```python
from build123d import *

# Parameters (mm, degrees)
F1_DEPTH = 7
F2_R     = 3.5
F3_DEPTH = 4
F5_DEPTH = 55
F7_DEPTH = 5


with BuildPart() as f1:
    # F0 (on Front) → F1 (new body)
    with BuildSketch(Plane.XZ):
        Polygon((12.5, 10), (0, 10), (-12.5, 10), (-12.5, 0.040646), (-12.5, -10), (12.5, -10), align=None)
    extrude(amount=F1_DEPTH)

    # F2 (on Front) → F3 (cut)
    with BuildSketch(Plane.XZ):
        Circle(F2_R)
    extrude(amount=F3_DEPTH, mode=Mode.SUBTRACT)

    # F4 (on face) → F5 (join)
    with BuildSketch(Plane.XZ.offset(7)):
        Polygon((2.5, 6.950472), (0, 6.950472), (-2.5, 6.950472), (-2.5, 1.950472), (2.5, 1.950472), align=None)
    extrude(amount=F5_DEPTH)

    # F6 (on face) → F7 (join)
    with BuildSketch(Plane.YZ.offset(2.5)):
        Polygon((-5.509801, -4.645343), (-18.229285, 1.950472), (-23.229285, 1.950472), (-5.509801, -8.645343), align=None)
    extrude(amount=-F7_DEPTH)


solid = f1.part
```
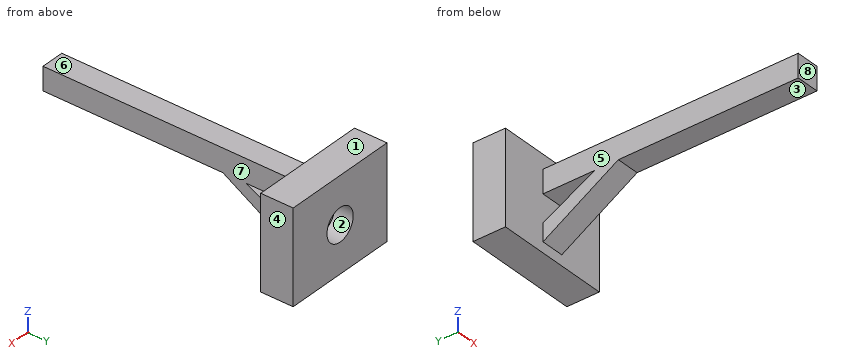
Design review of the part built by this model. Coordinates are the model's own, in mm. Face numbers are marked on the shaded views. A direction names the side the tool comes from. Give positions to 0.01 mm unless a question says otherwise; leave off trailing zeros. Loops run counter-clockwise (first coordinate to the right, second up) from the corner with the lowest first, then second, coordinate; pieces in that order, holes last. Notation, with made-up numbers: M 61.5,31 L 100.5,31 A7 ccw 100.5,37 Z; hole C -22,-22.75 d7. An arc over 180 degrees is marked long. Return JSON: item names as keys, results as strings. Group by question number.
Item 1: Mouldability with a two-part tool opening along Z and no side actions: class the marked faces 1, 2, 3 and 4 as released by +Z, released by -Z, zero draft, split by the parting line, or undercut.
Item 2: We need section C-C (x = 0). Give the boundary of the cut face in (y, z).
Item 3: We need section A-A (z = -1.5). Give the boundary of the cut face in (x, y), and give its area (3 significant figures).
Item 4: We need section D-D (y = -55.5). Give the boundary of the cut face in (x, z), and give its area (3 significant figures).
Item 5: Insertion check: pin 1 Ø7.5 at (y, z) = (-41.5, -3.5) entering from -X; pin 2 Ø2 at (x, y) = (1.5, -21.5) entering from -Z; pin 3 Ø10 at (x, y) = (4.5, -16.5) entering from +Z; pin 4 Ø1.5 at (x, y) = (1, -37) entering from -Z. Each pin has a flat end and moves straight along its axis. Give the tip position at first contact, or say it passes through.
Item 6: We need section B-B (y = -8). Give the boundary of the cut face in (x, z).
Item 7: For probe 1 along Z at (x, y) = (0, -2.55); probe 2 along Y at (x, z) = (7.5, 4.5); probe 3 along Z at (x, y) = (-1.5, -52), list the stretches that pass through material, from the lowest coordinate up.
Item 8: Tool access review of the marked faces 5, 6, 7 and 8: name each direction out of +Z, -Z, +X, -X, +Y, -Y from which nothing blocks a thin tool from reaching the whole face with its end or side.
Output:
{
 "1": {"face 1": "released by +Z", "face 2": "undercut", "face 3": "released by -Z", "face 4": "zero draft"},
 "2": {"outline": "M -62,1.95 L -23.23,1.95 L -7,-7.75 L -7,-10 L 0,-10 L 0,-3.5 L -4,-3.5 L -4,3.5 L 0,3.5 L 0,10 L -7,10 L -7,6.95 L -62,6.95 Z; hole M -18.23,1.95 L -7,-3.87 L -7,1.95 Z"},
 "3": {"outline": "M -12.5,-7 L 12.5,-7 L 12.5,0 L 3.16,0 L 3.16,-4 L -3.16,-4 L -3.16,0 L -12.5,0 Z; M -2.5,-17.46 L 2.5,-17.46 L 2.5,-11.58 L -2.5,-11.58 Z", "area": "179 mm^2"},
 "4": {"outline": "M -2.5,1.95 L 2.5,1.95 L 2.5,6.95 L -2.5,6.95 Z", "area": "25.0 mm^2"},
 "5": {"pin 1": "passes through", "pin 2": "stops at z = 0.32", "pin 3": "stops at z = 6.95", "pin 4": "stops at z = 1.95"},
 "6": {"outline": "M -2.5,-7.16 L 2.5,-7.16 L 2.5,-3.35 L -2.5,-3.35 Z; M -2.5,1.95 L 2.5,1.95 L 2.5,6.95 L -2.5,6.95 Z"},
 "7": {"probe 1": "z = -10 to -3.5, 3.5 to 10", "probe 2": "y = -7 to 0", "probe 3": "z = 1.95 to 6.95"},
 "8": {"face 5": "+Z, -Z, -X, -Y", "face 6": "+Z, +X, -X, -Y", "face 7": "+Z, -Z, +X, -Y", "face 8": "+Z, -Z, +X, -X, -Y"}
}
